from build123d import *

# Parameters (mm, degrees)
PILLOW_SKETCH_W                                  = 22
PILLOW_SKETCH_H                                  = 49
PILLOW_SKETCH_W_2                                = 11
BASE_BOSS_EXTRUDE_DEPTH                          = 27
PILLOW_SKETCH_4_W                                = 11
PILLOW_SKETCH_4_H                                = 49
THRUST_START                                     = -4
THRUST_BEARING_STACK_CUT_REVOLVE_DEPTH           = 23
THRUST_START_2                                   = -6.5
THRUST_BEARING_STACK_CUT_REVOLVE_2_DEPTH         = 28
PILLOW_SKETCH_6_W                                = 14
PILLOW_SKETCH_6_H                                = 1
CBORE_FOR_M3_PAN_HEAD_MACHINE_SCREW1_D           = 3.4
CBORE_FOR_M3_PAN_HEAD_MACHINE_SCREW1_CBORE_D     = 7
CBORE_FOR_M3_PAN_HEAD_MACHINE_SCREW1_CBORE_DEPTH = 24
STEPPER_PLATE_MOUNT_M5_CLEARANCE_HOLE_D          = 5.3


# Read off the part's stored shape, not the designer's step: Thrust Bearing Stack Cut-Revolve
with BuildPart() as part:
    # Pillow Sketch → Base Boss-Extrude (new body)
    with BuildSketch(Plane(origin=(0, 0, 0), x_dir=(1, 0, 0), z_dir=(0, 1, 0))):
        with Locations((-22, 0)):
            Rectangle(PILLOW_SKETCH_W, PILLOW_SKETCH_H)
        with Locations((-5.5, 0)):
            Rectangle(PILLOW_SKETCH_W_2, PILLOW_SKETCH_H)
    base_boss_extrude = extrude(amount=-BASE_BOSS_EXTRUDE_DEPTH)

    # Pillow Sketch<4> → Shaft Clearance Cut-Revolve (revolve, cut)
    with BuildSketch(Plane(origin=(0, 0, 0), x_dir=(1, 0, 0), z_dir=(0, 1, 0))):
        with Locations((-5.5, 0)):
            Rectangle(PILLOW_SKETCH_4_W, PILLOW_SKETCH_4_H)
    shaft_clearance_cut_revolve = revolve(axis=Axis((0, 0, -24.5), (0, 0, 1)), mode=Mode.SUBTRACT)

    # Thrust Bearing Stack Cut-Revolve outline → Thrust Bearing Stack Cut-Revolve (cut)
    with BuildSketch(Plane.XY.offset(THRUST_START)):
        with BuildLine():
            ThreePointArc((-24, 0), (-16.970562748, -16.970562748), (0, -24))
            Line((0, -24), (0, -11))
            ThreePointArc((0, -11), (-7.778174593, -7.778174593), (-11, 0))
            Line((-11, 0), (-24, 0))
        make_face()
    thrust_bearing_stack_cut_revolve = extrude(amount=THRUST_BEARING_STACK_CUT_REVOLVE_DEPTH, mode=Mode.SUBTRACT)

    # Thrust Bearing Stack Cut-Revolve 2 outli → Thrust Bearing Stack Cut-Revolve 2 (cut)
    with BuildSketch(Plane.XY.offset(THRUST_START_2)):
        with BuildLine():
            ThreePointArc((-17.5, 0), (-12.374368671, -12.374368671), (0, -17.5))
            Line((0, -17.5), (0, -11))
            ThreePointArc((0, -11), (-7.778174593, -7.778174593), (-11, 0))
            Line((-11, 0), (-17.5, 0))
        make_face()
    thrust_bearing_stack_cut_revolve_2 = extrude(amount=THRUST_BEARING_STACK_CUT_REVOLVE_2_DEPTH, mode=Mode.SUBTRACT)

    # Pillow Sketch<6> → Rotary Bearing Cut-Revolve (revolve, cut)
    with BuildSketch(Plane(origin=(0, 0, 0), x_dir=(1, 0, 0), z_dir=(0, 1, 0))):
        Polygon((14, 21), (0, 21), (0, 12), (14, 12), (18.5, 12), (18.5, 21), align=None)
        with Locations((7, 21.5)):
            Rectangle(PILLOW_SKETCH_6_W, PILLOW_SKETCH_6_H)
        with Locations((7, 11.5)):
            Rectangle(PILLOW_SKETCH_6_W, PILLOW_SKETCH_6_H)
    rotary_bearing_cut_revolve = revolve(axis=Axis((0, 0, -24.5), (0, 0, 1)), mode=Mode.SUBTRACT)

    # CBORE for M3 Pan Head Machine Screw1 (through all)
    with Locations(Plane(origin=(0, -27, 0), x_dir=(-1, 0, 0), z_dir=(0, -1, 0))):
        with Locations((29, -20.5), (29, -10.25), (29, 0), (29, 10.25), (29, 20.5)):
            cbore_for_m3_pan_head_machine_screw1 = CounterBoreHole(CBORE_FOR_M3_PAN_HEAD_MACHINE_SCREW1_D / 2, CBORE_FOR_M3_PAN_HEAD_MACHINE_SCREW1_CBORE_D / 2, CBORE_FOR_M3_PAN_HEAD_MACHINE_SCREW1_CBORE_DEPTH)

    # Cover Mirror: Base Boss-Extrude, Shaft Clearance Cut-Revolve, Thrust Bearing Stack Cut-Revolve, Thrust Bearing Stack Cut-Revolve 2, Rotary Bearing Cut-Revolve, CBORE for M3 Pan Head Machine Screw1 across plane
    add(base_boss_extrude.mirror(Plane(origin=(0, 0, 0), x_dir=(0, 0, 1), z_dir=(1, 0, 0))))
    add(shaft_clearance_cut_revolve.mirror(Plane(origin=(0, 0, 0), x_dir=(0, 0, 1), z_dir=(1, 0, 0))), mode=Mode.SUBTRACT)
    add(thrust_bearing_stack_cut_revolve.mirror(Plane(origin=(0, 0, 0), x_dir=(0, 0, 1), z_dir=(1, 0, 0))), mode=Mode.SUBTRACT)
    add(thrust_bearing_stack_cut_revolve_2.mirror(Plane(origin=(0, 0, 0), x_dir=(0, 0, 1), z_dir=(1, 0, 0))), mode=Mode.SUBTRACT)
    add(rotary_bearing_cut_revolve.mirror(Plane(origin=(0, 0, 0), x_dir=(0, 0, 1), z_dir=(1, 0, 0))), mode=Mode.SUBTRACT)
    add(cbore_for_m3_pan_head_machine_screw1.mirror(Plane(origin=(0, 0, 0), x_dir=(0, 0, 1), z_dir=(1, 0, 0))), mode=Mode.SUBTRACT)

    # Stepper Plate Mount M5 Clearance Hole (through all)
    with Locations(Plane.XY.offset(24.5)):
        with Locations((-20, -22.360679775), (20, -22.360679775)):
            Hole(STEPPER_PLATE_MOUNT_M5_CLEARANCE_HOLE_D / 2)


solid = part.part
Part model, mm, in its own coordinate system. A direction names the side the tool comes from. Round coordinates to 2 decimals unless told otherwise and drop trailing zeros. Write each loop counter-clockwise with the first axis right and the second up, starting at its lowest first coordinate (ties: lowest second). Pieces come first, ordered by that corner, then holes. Notation, with made-up numbers: M 64,52.5 L 117,52.5 A13 ccw 117,71.5 Z; hole C 28.25,85.25 d1. An arc over 180 degrees is marked long. Return JSON: item names as keys, results as strings. Group by question number.
(1) Saw through at D-D on x = 5. Write the cut outline in (y, z), then the cut area to 3 significant figures.
(2) Pin check, flat tip, straight feed: pin 1 Ø4 at (x, z) = (29, 10.25) entering from -Y. Stop position of the tip, or through.
(3) Drill centre lines: probe 1 along Z at (x, y) = (-29, -14.25); probe 2 along X at (y, z) = (-19.5, -20.5); probe 3 along X at (y, z) = (-16.75, -11.5). Where is each one in solid material? Low to high.
(4) Saw through at B-B on z = 9.5. Write the cut outline in (x, y), then the cut area to 3 significant figures.
(5) Which spindle directions (+Z, -Z, +X, -X, +Y, -Y) get a long thin tool onto all of the face, cutting with end or side? Do faces 5 (the face through (0, -13, -24.5)), 6 (the face through (32.34, -15.17, -1.05)). Say none if no direction does.
(6) Saw through at A-A on x = -20. Write the cut outline in (y, z).
(7) Two-plate mould, pull along X, no slides. Class faces 1 (the face through (-31, -3, -11)), 2 (the face through (-33, -13, 0)), 3 (the face through (0, -27, 0)), 4 (the face through (27.38, -1.48, -0.51)): +X half, -X half, draft (parallel to the pull), parting line (faces both ways), or undercut.
(8) Saw through at C-C on z = -16. Write the cut outline in (x, y), then the cut area to 3 significant figures.
Returned:
{
 "1": {"outline": "M -27,-24.5 L -9.8,-24.5 L -9.8,-22 L -13.08,-22 L -13.08,-21 L -17.81,-21 L -17.81,-12 L -13.08,-12 L -13.08,-11 L -9.8,-11 L -9.8,-6.5 L -16.77,-6.5 L -16.77,-4 L -23.47,-4 L -23.47,19 L -16.77,19 L -16.77,21.5 L -9.8,21.5 L -9.8,24.5 L -27,24.5 Z", "area": "415 mm²"},
 "2": {"pin 1": "y = -3"},
 "3": {"probe 1": "-24.5 to -24, -17 to -13.75, -6.75 to -3.5, 3.5 to 6.75, 13.75 to 17, 24 to 24.5", "probe 2": "-33 to -32.5, -25.5 to 25.5, 32.5 to 33", "probe 3": "-33 to -32.27, -25.73 to 25.73, 32.27 to 33"},
 "4": {"outline": "M -33,-27 L -32.42,-27 L -32.42,-3 L -30.53,-3 L -30.53,0 L -33,0 Z; M -27.47,-3 L -25.58,-3 L -25.58,-27 L 25.58,-27 L 25.58,-3 L 27.47,-3 L 27.47,0 L 24,0 A24 cw -24,0 L -27.47,0 Z; M 30.53,-3 L 32.42,-3 L 32.42,-27 L 33,-27 L 33,0 L 30.53,0 Z; hole C -20,-22.36 d5.3; hole C 20,-22.36 d5.3", "area": "487 mm²"},
 "5": {"face 5": "-Z, +X, -X, +Y, -Y", "face 6": "-Y"},
 "6": {"outline": "M -27,-24.5 L -25.01,-24.5 L -25.01,24.5 L -27,24.5 Z; M -19.71,-24.5 L 0,-24.5 L 0,-4 L -13.27,-4 L -13.27,19 L 0,19 L 0,24.5 L -19.71,24.5 Z"},
 "7": {"face 1": "undercut", "face 2": "-X half", "face 3": "draft", "face 4": "undercut"},
 "8": {"outline": "M -33,-27 L 33,-27 L 33,0 L 18.5,0 A18.5 cw -18.5,0 L -33,0 Z; hole C -20,-22.36 d5.3; hole C 20,-22.36 d5.3", "area": "1,200 mm²"}
}
